Job drawing, mm, ordinate dimensions from the low corner. One solid piece. A direction names the side the tool comes from. Coordinates: 2 decimals unless noted, no trailing zeros. Write each loop counter-clockwise with the first axis right and the second up, starting at its lowest first coordinate (ties: lowest second). Pieces come first, ordered by that corner, then holes.
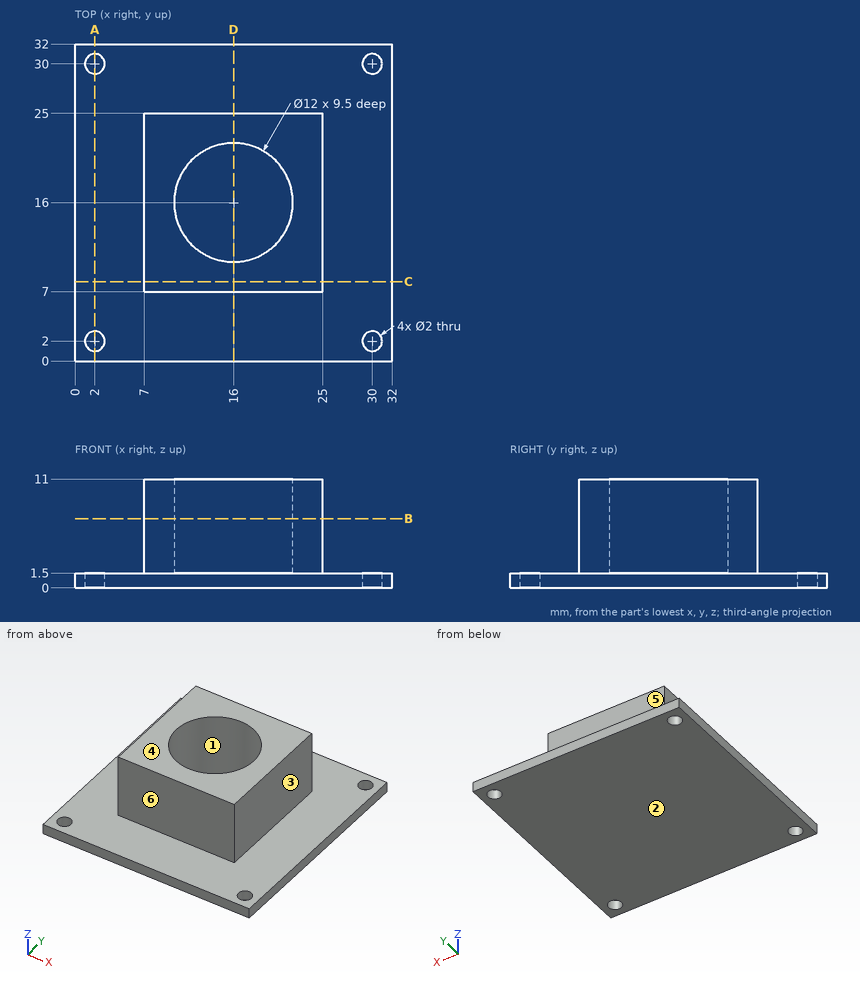
1. Saw through at A-A on x = 2. List the corners of the cut face in (y, z).
Computed values:
outline: (0, 0) - (1, 0) - (1, 1.5) - (0, 1.5) - close; (3, 0) - (29, 0) - (29, 1.5) - (3, 1.5) - close; (31, 0) - (32, 0) - (32, 1.5) - (31, 1.5) - close
2. Probe line 1 along Y through (x, z) = (2, 1.1); line 2 along Y through (x, z) = (16, 4); line 3 along Z through (x, y) = (5, 29). List the from-to ranges inside material, lowest first.
Computed values:
line 1: y = 0 to 1, 3 to 29, 31 to 32
line 2: y = 7 to 10, 22 to 25
line 3: z = 0 to 1.5
3. Flat gauge pins, fed straight in: pin 1 (2 mm diameter, centred on x = 21, z = 6, fed in from +Y); pin 2 (3.5 mm diameter, centred on x = 14, y = 13, fed in from +Z); pin 3 (5 mm diameter, centred on y = 17, z = 7, fed in from -X). Where does each tip first touch, or does it go through?
Computed values:
pin 1: stops at y = 25
pin 2: stops at z = 1.5
pin 3: stops at x = 7
4. 3-axis set-ups, long thin cutter, end or side, ignore diameter. For the marked faces 4, 5 and 6: which of +Z, -Z, +X, -X, +Y, -Y reach the whole face in a straight line?
Computed values:
face 4: +Z, +X, -X, +Y, -Y
face 5: +Z, +X, -X, +Y
face 6: +Z, +X, -X, -Y
5. Saw through at D-D on x = 16. List the corners of the cut face in (y, z), plus the area to 3 significant figures.
Computed values:
outline: (0, 0) - (32, 0) - (32, 1.5) - (25, 1.5) - (25, 11) - (22, 11) - (22, 1.5) - (10, 1.5) - (10, 11) - (7, 11) - (7, 1.5) - (0, 1.5) - close
area: 105 mm2
6. Saw through at B-B on z = 7. List the corners of the cut face in (x, y), plus the area to 3 significant figures.
Computed values:
outline: (7, 7) - (25, 7) - (25, 25) - (7, 25) - close; hole circle Ø12 at (16, 16)
area: 211 mm2
7. Mould opens along X. For the marked faces 1, 2 and 3 say: +X half, -X half, draft (parallel to the pull), parting line (faces both ways), or undercut.
Computed values:
face 1: undercut
face 2: draft
face 3: +X half
8. Saw through at C-C on y = 8. List the corners of the cut face in (x, z).
Computed values:
outline: (0, 0) - (32, 0) - (32, 1.5) - (25, 1.5) - (25, 11) - (7, 11) - (7, 1.5) - (0, 1.5) - close
